```python
from build123d import *

# Parameters (mm, degrees)
SKETCH1_W         = 36
SKETCH1_H         = 63
SKETCH1_W_2       = 32
SKETCH1_H_2       = 59
WALL_HEIGHT_DEPTH = 20
ROOF_START        = 20
SKETCH1_3_W       = 36
SKETCH1_3_H       = 63
SKETCH1_3_W_2     = 32
SKETCH1_3_H_2     = 59
ROOF_DEPTH        = 2


with BuildPart() as part:
    # Sketch1 → Wall_Height (new body)
    with BuildSketch(Plane.XY):
        with Locations((18, -31.5)):
            Rectangle(SKETCH1_W, SKETCH1_H)
        with Locations((18, -31.5)):
            Rectangle(SKETCH1_W_2, SKETCH1_H_2, mode=Mode.SUBTRACT)
    extrude(amount=WALL_HEIGHT_DEPTH)

    # Sketch1<3> → Roof (add)
    # profile 1 of 2: a face of its own
    with BuildSketch(Plane.XY.offset(ROOF_START)):
        with Locations((18, -31.5)):
            Rectangle(SKETCH1_3_W, SKETCH1_3_H)
        with Locations((18, -31.5)):
            Rectangle(SKETCH1_3_W_2, SKETCH1_3_H_2, mode=Mode.SUBTRACT)
    # profile 2 of 2: a face of its own
    with BuildSketch(Plane.XY.offset(ROOF_START)):
        with Locations((18, -31.5)):
            Rectangle(SKETCH1_3_W_2, SKETCH1_3_H_2)
    extrude(amount=ROOF_DEPTH)


solid = part.part
```
The model under review builds one solid part; all positions refer to its coordinate system, in mm. A direction names the side the tool comes from. Coordinates: 2 decimals unless noted, no trailing zeros. Write each loop counter-clockwise with the first axis right and the second up, starting at its lowest first coordinate (ties: lowest second). Pieces come first, ordered by that corner, then holes.
1) We need section C-C on y = -45. State the section outline as (x, z) points.
2) To check wall thickness, follow probe 1 along X at (y, z) = (-50, 8.5); probe 2 along Y at (x, z) = (4, 1.25); probe 3 along Z at (x, y) = (31, -22.5). State the ranges of each line that lie inside material, in increasing order.
3) We need section A-A on z = 11.25. State the section outline as (x, y) points, then the cut area to 3 significant figures.
4) Machinability: for faces 5 (the face through (18, -61, 10)), 6 (the face through (18, -31, 22)), which of the approach directions +Z, -Z, +X, -X, +Y, -Y give a long, thin tool a straight path to every point of the face, cutting with its end or side? Answer none if there is none.
5) The part is to be moulded in two halves that separate along X. For faces 1 (the face through (0, -32, 11)), 2 (the face through (18, -31, 20)), 3 (the face through (2, -32, 10)), 4 (the face through (18, -63, 11)), say which applies: pulls with the +X half, pulls with the -X half, needs draft (parallel to the pull), parting line crosses it, or undercut.
6) Clearance check with a flat-ended pin moving along its axis: pin 1 Ø9.5 at (x, y) = (10.5, -35.5) entering from -Z. State where the tip first meets the part, or that it passes through.
7) We need section B-B on x = 17. State the section outline as (y, z) points, then the cut area to 3 significant figures.
Answer list:
1. outline: (0, 0) - (2, 0) - (2, 20) - (34, 20) - (34, 0) - (36, 0) - (36, 22) - (0, 22) - close
2. probe 1: x = 0 to 2, 34 to 36
2. probe 2: y = -63 to -61, -2 to 0
2. probe 3: z = 20 to 22
3. outline: (0, -63) - (36, -63) - (36, 0) - (0, 0) - close; hole (2, -61) - (34, -61) - (34, -2) - (2, -2) - close
3. area: 380 mm2
4. face 5: -Z
4. face 6: +Z, +X, -X, +Y, -Y
5. face 1: pulls with the -X half
5. face 2: undercut
5. face 3: undercut
5. face 4: needs draft
6. pin 1: stops at z = 20
7. outline: (-63, 0) - (-61, 0) - (-61, 20) - (-2, 20) - (-2, 0) - (0, 0) - (0, 22) - (-63, 22) - close
7. area: 206 mm2
